Build history of the part. All positions in model axes, mm. Face numbers are marked on the shaded views. Coordinates: 2 decimals unless noted, no trailing zeros. Order: outer loops, then holes, each group sorted by start corner. A loop starts at its lowest first (then second) coordinate and runs counter-clockwise, first axis right, second up. Notation, with made-up numbers: (-28, 17) - (29, 17) arc R15 cw to (29, 36) - close; hole circle Ø10 at (-34, -30.75). An arc over 180 degrees is marked (long way). Answer as CSV lines item,"result". Start each with the question number.
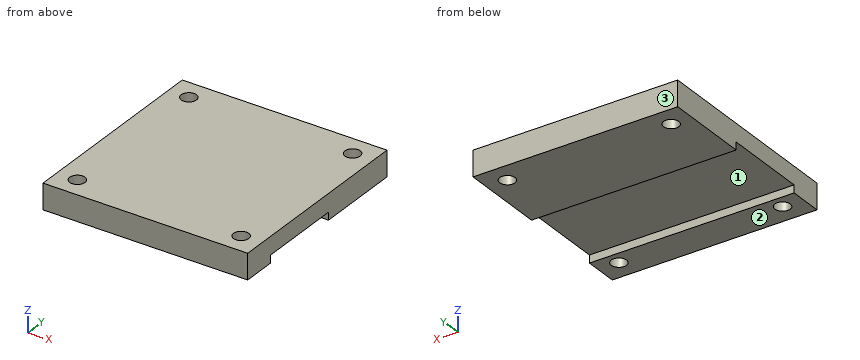
from build123d import *

# Parameters (mm, degrees)
SKETCH1_W           = 40
SKETCH1_H           = 40
SKETCH1_R           = 1.5
BOSS_EXTRUDE1_DEPTH = 5
SKETCH3_W           = 40
SKETCH3_H           = 16.636061704
CUT_EXTRUDE1_DEPTH  = 1.5


with BuildPart() as part:
    # Sketch1 → Boss-Extrude1 (new body)
    with BuildSketch(Plane.XY):
        Rectangle(SKETCH1_W, SKETCH1_H)
        with Locations((-16, 16)):
            Circle(SKETCH1_R, mode=Mode.SUBTRACT)
        with Locations((16, 16)):
            Circle(SKETCH1_R, mode=Mode.SUBTRACT)
        with Locations((-16, -16)):
            Circle(SKETCH1_R, mode=Mode.SUBTRACT)
        with Locations((16, -16)):
            Circle(SKETCH1_R, mode=Mode.SUBTRACT)
    extrude(amount=BOSS_EXTRUDE1_DEPTH)

    # Sketch3 → Cut-Extrude1 (cut)
    with BuildSketch(Plane(origin=(0, 0, 0), x_dir=(-1, 0, 0), z_dir=(0, 0, -1))):
        with Locations((0, -5.111977567)):
            Rectangle(SKETCH3_W, SKETCH3_H)
    extrude(amount=-CUT_EXTRUDE1_DEPTH, mode=Mode.SUBTRACT)


solid = part.part
(1) Band-saw the part on B-B on x = 16. List the corners of the cut face in (y, z), plus the area to 3 significant figures.
(2) Probe L1, parallel to Y at x = 16, z = 2; L2, parallel to X at y = -16.5, z = 0.4; L3, parallel to Y at x = 18, z = 1.4. List the from-to ranges inside material, lowest first. Write a range as [from, to].
(3) Band-saw the part on A-A on y = 16. List the corners of the cut face in (x, z), plus the area to 3 significant figures.
(4) Pull direction Y, two halves, no side cores. Call the marked faces 1, 2 and 3: +Y half, -Y half, draft (parallel to the pull), parting line (faces both ways), or undercut.
(5) Band-saw the part on C-C on z = 3.15. List the corners of the cut face in (x, y).
(6) Band-saw the part on D-D on x = -13.5. List the corners of the cut face in (y, z).
(7) Drop a flat-ended pin along its axis: pin 1 Ø5 at (x, y) = (-6.5, -6) entering from -Z. Give the stop position or say it passes through.
Filled in:
1,outline,"(-20, 0) - (-17.5, 0) - (-17.5, 5) - (-20, 5) - close; (-14.5, 0) - (-13.43, 0) - (-13.43, 1.5) - (3.21, 1.5) - (3.21, 0) - (14.5, 0) - (14.5, 5) - (-14.5, 5) - close; (17.5, 0) - (20, 0) - (20, 5) - (17.5, 5) - close"
1,area,"145 mm^2"
2,L1,"y = [-20, -17.5], [-14.5, 14.5], [17.5, 20]"
2,L2,"x = [-20, -17.41], [-14.59, 14.59], [17.41, 20]"
2,L3,"y = [-20, -13.43], [3.21, 20]"
3,outline,"(-20, 0) - (-17.5, 0) - (-17.5, 5) - (-20, 5) - close; (-14.5, 0) - (14.5, 0) - (14.5, 5) - (-14.5, 5) - close; (17.5, 0) - (20, 0) - (20, 5) - (17.5, 5) - close"
3,area,"170 mm^2"
4,face 1,"undercut"
4,face 2,"draft"
4,face 3,"+Y half"
5,outline,"(-20, -20) - (20, -20) - (20, 20) - (-20, 20) - close; hole circle Ø3 at (-16, -16); hole circle Ø3 at (-16, 16); hole circle Ø3 at (16, -16); hole circle Ø3 at (16, 16)"
6,outline,"(-20, 0) - (-13.43, 0) - (-13.43, 1.5) - (3.21, 1.5) - (3.21, 0) - (20, 0) - (20, 5) - (-20, 5) - close"
7,pin 1,"stops at z = 1.5"
